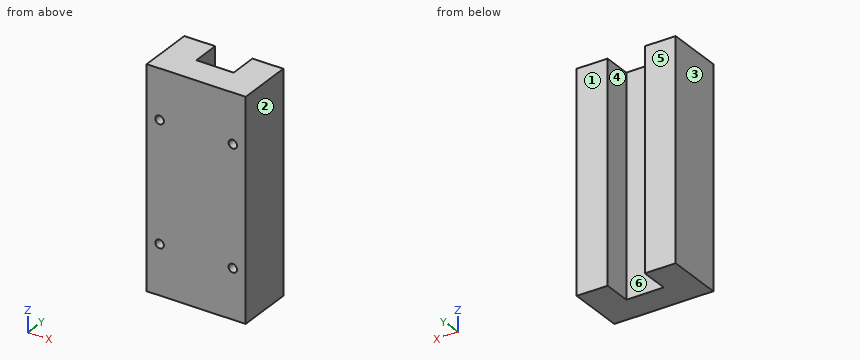
Autodesk Inventor part; units mm, degrees
ref_plane "YZ Plane" through (0, 0, 0) normal (1, 0, 0) x (0, 1, 0)
ref_plane "XZ Plane" through (0, 0, 0) normal (0, 1, 0) x (-1, 0, 0)
ref_plane "XY Plane" through (0, 0, 0) normal (0, 0, 1) x (1, 0, 0)
sketch "Sketch1" plane through (0, 0, 0) normal (0, 0, 1) x (1, 0, 0)
  line L0 (7.6927, 4.9102) -> (7.6927, -20.4898)
  line L1 (7.6927, -20.4898) -> (-36.7573, -20.4898)
  line L2 (-36.7573, -20.4898) -> (-36.7573, 4.9102)
  line L3 (-6.1503, 2.7687) -> (-6.1503, -7.7898)
  line L4 (-6.1503, -7.7898) -> (-22.9143, -7.7898)
  line L5 (-22.9143, -7.7898) -> (-22.9143, 2.7687)
  line L6 (-22.9143, 2.7687) -> (-22.9143, 4.9102)
  line L7 (-6.1503, 2.7687) -> (-6.1503, 4.9102)
  line L8 (-36.7573, 4.9102) -> (-22.9143, 4.9102)
  line L9 (-6.1503, 4.9102) -> (7.6927, 4.9102)
  point P0 (0, 0)
  dimension "d0" = 44.45
  dimension "d1" = 25.4
  dimension "d2" = 16.764
  dimension "d4" = 13.843
  dimension "d5" = 13.843
  dimension "d6" = 12.7
extrude "Extrusion1" add sketch "Sketch1" along normal blind 97.917
sketch "Sketch2" plane through (-36.7573, -20.4898, 0) normal (0, -1, 0) x (1, 0, 0)
  line L0 (44.45, 0) -> (44.45, 97.917)
  line L1 (0, 0) -> (0, 97.917)
  line L2 (0, 0) -> (44.45, 0)
  line L3 (0, 97.917) -> (44.45, 97.917)
  point P0 (36.7573, 0)
  point P1 (38.6715, 22.225)
  point P2 (5.7785, 22.225)
  point P3 (5.7785, 75.692)
  point P4 (38.6715, 75.692)
  dimension "d9" = 5.7785
  dimension "d10" = 5.7785
  dimension "d11" = 22.225
  dimension "d12" = 22.225
  dimension "d13" = 5.7785
  dimension "d14" = 5.7785
  dimension "d15" = 22.225
  dimension "d16" = 22.225
  dimension "d17" = 53.467
  dimension "d18" = 53.467
hole "Hole1" at (1.9142, -20.4898, 22.225) at (-30.9788, -20.4898, 22.225) at (-30.9788, -20.4898, 75.692) at (1.9142, -20.4898, 75.692) direction (0, 1, 0) diameter 3.81 depth 7.62
properties part number "Rail Slider"
CAD build for the part. Positions are in the model's coordinates, mm. Face numbers are marked on the shaded views. A direction names the side the tool comes from. Round coordinates to 2 decimals unless told otherwise and drop trailing zeros. Write each loop counter-clockwise with the first axis right and the second up, starting at its lowest first coordinate (ties: lowest second). Pieces come first, ordered by that corner, then holes. Notation, with made-up numbers: (77, -30) -> (132, -30) arc R31 cw to (132, 5) -> close; hole circle Ø8 at (50.25, -4). An arc over 180 degrees is marked (long way). Answer in a Markdown table with one row per item. Add a question column.
Item 1: Mould opens along X. For the marked faces 1, 2, 3 and 4 say: pulls with the +X half, pulls with the -X half, needs draft (parallel to the pull), parting line crosses it, or undercut.
Item 2: Saw through at C-C, the plane x = -30. Write the cut outline in (y, z).
Item 3: Saw through at A-A, the plane y = -3. Write the cut outline in (x, z).
Item 4: Saw through at D-D, the plane z = 23. Write the cut outline in (x, y).
Item 5: Saw through at B-B, the plane z = 64.5. Write the cut outline in (x, y).
Item 6: Which spindle directions (+Z, -Z, +X, -X, +Y, -Y) get a long thin tool onto all of the face, cutting with end or side? Do the marked faces 5 and 6. Say none if no direction does.
Item 7: Drop flat-ended pins along their axis: pin 1 Ø3 at (x, z) = (1.5, 76) entering from -Y; pin 2 Ø1 at (x, y) = (-7.5, -5.5) entering from -Z; pin 3 Ø1.9 at (x, z) = (-30.5, 23) entering from -Y. Give the stop position or say it passes through.
Item 8: Drill centre lines: line 1 (X direction, y = 4, z = 32); line 2 (Y direction, x = -12.5, z = 41). Where is each one in solid material? Low to high. Write a range as from..to.
Findings below:
| question | item | result |
|---|---|---|
| 1 | face 1 | needs draft |
| 1 | face 2 | pulls with the +X half |
| 1 | face 3 | pulls with the -X half |
| 1 | face 4 | undercut |
| 2 | outline | (-20.49, 0) -> (4.91, 0) -> (4.91, 97.92) -> (-20.49, 97.92) -> (-20.49, 77.33) -> (-12.87, 77.33) -> (-12.87, 74.06) -> (-20.49, 74.06) -> (-20.49, 23.86) -> (-12.87, 23.86) -> (-12.87, 20.59) -> (-20.49, 20.59) -> close |
| 3 | outline | (-36.76, 0) -> (-22.91, 0) -> (-22.91, 97.92) -> (-36.76, 97.92) -> close; (-6.15, 0) -> (7.69, 0) -> (7.69, 97.92) -> (-6.15, 97.92) -> close |
| 4 | outline | (-36.76, -20.49) -> (-32.72, -20.49) -> (-32.72, -12.87) -> (-29.24, -12.87) -> (-29.24, -20.49) -> (0.17, -20.49) -> (0.17, -12.87) -> (3.65, -12.87) -> (3.65, -20.49) -> (7.69, -20.49) -> (7.69, 4.91) -> (-6.15, 4.91) -> (-6.15, -7.79) -> (-22.91, -7.79) -> (-22.91, 4.91) -> (-36.76, 4.91) -> close |
| 5 | outline | (-36.76, -20.49) -> (7.69, -20.49) -> (7.69, 4.91) -> (-6.15, 4.91) -> (-6.15, -7.79) -> (-22.91, -7.79) -> (-22.91, 4.91) -> (-36.76, 4.91) -> close |
| 6 | face 5 | +Z, -Z, +X, -X, +Y |
| 6 | face 6 | +Z, -Z, +Y |
| 7 | pin 1 | stops at y = -20.49 |
| 7 | pin 2 | passes through |
| 7 | pin 3 | stops at y = -12.87 |
| 8 | line 1 | x = -36.76..-22.91, -6.15..7.69 |
| 8 | line 2 | y = -20.49..-7.79 |
